from build123d import *

# Parameters (mm, degrees)
F0_W      = 56.902528
F0_H      = 72.428972
F1_DEPTH  = 28.647777
F2_R      = 25.4
F1_FACE_W = 6.102528
F1_FACE_H = 6.495554
F3_DEPTH  = 139.845217


with BuildPart() as f1:
    # F0 (on Top) → F1 (new body, symmetric)
    with BuildSketch(Plane.XY):
        with Locations((28.451264, -36.214486)):
            Rectangle(F0_W, F0_H)
    extrude(amount=F1_DEPTH, both=True)

    # F2
    f2_edges = [f1.edges().sort_by_distance(p)[0] for p in [
        (56.902528, 0, 0),
        (28.451264, 0, -28.647777),
        (0, 0, 0),
        (28.451264, 0, 28.647777),
    ]]
    fillet(f2_edges, radius=F2_R)

    # F1_face (on face) → F3 (join)
    with BuildSketch(Plane(origin=(28.451264, 0, 0), x_dir=(-1, 0, 0), z_dir=(0, 1, 0))):
        Rectangle(F1_FACE_W, F1_FACE_H)
    extrude(amount=F3_DEPTH)


solid = f1.part
CAD build for the part. Positions are in the model's coordinates, mm. A direction names the side the tool comes from. Give positions to 0.01 mm unless a question says otherwise; leave off trailing zeros. Write each loop counter-clockwise with the first axis right and the second up, starting at its lowest first coordinate (ties: lowest second). Pieces come first, ordered by that corner, then holes. Notation, with made-up numbers: (15.25, 35.25) -> (47.25, 35.25) arc R8 ccw to (47.25, 50.25) -> close; hole circle Ø2 at (-33, 9.25). An arc over 180 degrees is marked (long way). Return JSON: item names as keys, results as strings.
Item 1: Drop flat-ended pins along their axis: pin 1 (3 mm diameter, centred on y = 64, z = 1.5, fed in from -X); pin 2 (2 mm diameter, centred on x = 34, z = -10, fed in from +Y); pin 3 (10 mm diameter, centred on x = 35.5, z = 9.5, fed in from +Y). Give the stop position or say it passes through.
Answer below:
{"pin 1": "stops at x = 25.4", "pin 2": "stops at y = -0.66", "pin 3": "stops at y = -0.06"}
Item 2: Band-saw the part on D-D (x = 17.5). List the corners of the cut face in (y, z).
Answer below:
{"outline": "(-72.43, -28.65) -> (-25.4, -28.65) arc R25.4 ccw to (-1.26, -11.15) -> (-1.26, 11.15) arc R25.4 ccw to (-25.4, 28.65) -> (-72.43, 28.65) -> close"}
Item 3: Band-saw the part on C-C (y = 9.5). List the corners of the cut face in (x, z).
Answer below:
{"outline": "(25.4, -3.25) -> (31.5, -3.25) -> (31.5, 3.25) -> (25.4, 3.25) -> close"}
Item 4: Band-saw the part on B-B (x = 45). List the corners of the cut face in (y, z).
Answer below:
{"outline": "(-72.43, -28.65) -> (-25.4, -28.65) arc R25.4 ccw to (-3.88, -16.75) -> (-3.88, 16.75) arc R25.4 ccw to (-25.4, 28.65) -> (-72.43, 28.65) -> close"}
Item 5: Band-saw the part on A-A (z = 1). List the corners of the cut face in (x, y).
Answer below:
{"outline": "(0, -72.43) -> (56.9, -72.43) -> (56.9, -25.4) arc R25.4 ccw to (31.5, 0) -> (31.5, 139.85) -> (25.4, 139.85) -> (25.4, 0) arc R25.4 ccw to (0, -25.4) -> close"}
Item 6: Drill centre lines: probe 1 along X at (y, z) = (28, -1); probe 2 along Y at (x, z) = (22, 18); probe 3 along Y at (x, z) = (11.5, 0). Where is each one in solid material? Low to high.
Answer below:
{"probe 1": "x = 25.4 to 31.5", "probe 2": "y = -72.43 to -4.72", "probe 3": "y = -72.43 to -4.14"}
Item 7: Tool access for faces 1 (the flat face through (28, -49, -28.648)), 2 (the flat face through (31.503, 69, 0)), 3 (the flat face through (28, 69, -3.248)), 4 (the flat face through (25.4, 69, 0)), 5 (the flat face through (28, 69, 3.248)): list every direction of +Z, -Z, +X, -X, +Y, -Y with a clear straight run to the whole face (end or side of a thin tool).
Answer below:
{"face 1": "-Z, +X, -X, +Y, -Y", "face 2": "+Z, -Z, +X, +Y", "face 3": "-Z, +X, -X, +Y", "face 4": "+Z, -Z, -X, +Y", "face 5": "+Z, +X, -X, +Y"}
